For this review, take the finished solid that the model builds, in its own axes (mm). A direction names the side the tool comes from. Coordinates: 2 decimals unless noted, no trailing zeros. Order: outer loops, then holes, each group sorted by start corner. A loop starts at its lowest first (then second) coordinate and runs counter-clockwise, first axis right, second up. Notation, with made-up numbers: (26, 48.5) -> (71, 48.5) arc R34 ccw to (71, 85.5) -> close; hole circle Ø11 at (-27.5, 48.25). An arc over 180 degrees is marked (long way). Write item = value, one per line. Start each with the question number.
1) Wall thickness on probe 1 along X at (y, z) = (1.5, 0.85); probe 2 along Y at (x, z) = (-3.5, 0.7): over which ranges is each line inside the solid? List them lowest first. Write a range as [from, to].
2) Consider section C-C on y = -6. Give the boundary of the cut face in (x, z).
3) Consider section A-A on z = 1.2. Give the boundary of the cut face in (x, y).
4) Draft analysis for pull direction Y (two halves, no side actions). For faces 3 (the face through (0, 20, 1)), 4 (the face through (-9, -15, 1)), 5 (the face through (0, -16, 1)), 6 (the face through (-20, 0, 1)), state which applies: +Y half, -Y half, draft (parallel to the pull), parting line (faces both ways), or undercut.
5) Machinability: for faces 1 (the face through (-15, -9, 1)), 2 (the face through (0, -20, 1)), which of the approach directions +Z, -Z, +X, -X, +Y, -Y give a long, thin tool a straight path to every point of the face, cutting with its end or side? Answer none if there is none.
6) Insertion check: pin 1 Ø8 at (x, y) = (1, 15.5) entering from -Z. The pin has a flat end and moves straight along its axis. Give the tip position at first contact, or say it passes through.
7) Consider section B-B on x = -6. Give the boundary of the cut face in (y, z), and give its area (3 significant figures).
from build123d import *

# Parameters (mm, degrees)
F0_W     = 40
F0_H     = 40
F0_W_2   = 18
F0_H_2   = 2
F0_W_3   = 2
F0_H_3   = 18
F1_DEPTH = 3
F2_R     = 2


with BuildPart() as f1:
    # F0 (on Top) → F1 (new body)
    with BuildSketch(Plane.XY):
        Rectangle(F0_W, F0_H)
        with Locations((0, -15)):
            Rectangle(F0_W_2, F0_H_2, mode=Mode.SUBTRACT)
        with Locations((-15, 0)):
            Rectangle(F0_W_3, F0_H_3, mode=Mode.SUBTRACT)
        with Locations((15, 0)):
            Rectangle(F0_W_3, F0_H_3, mode=Mode.SUBTRACT)
    extrude(amount=F1_DEPTH)

    # F2
    f2_edges = [f1.edges().sort_by_distance(p)[0] for p in [
        (20, -20, 1.5),
        (-20, -20, 1.5),
        (-20, 20, 1.5),
        (20, 20, 1.5),
    ]]
    fillet(f2_edges, radius=F2_R)


solid = f1.part
Answer sheet:
q1.probe_1 = [-20, -16], [-14, 14], [16, 20]
q1.probe_2 = [-20, -16], [-14, 20]
q2.outline = (-20, 0) -> (-16, 0) -> (-16, 3) -> (-20, 3) -> close; (-14, 0) -> (14, 0) -> (14, 3) -> (-14, 3) -> close; (16, 0) -> (20, 0) -> (20, 3) -> (16, 3) -> close
q3.outline = (-20, -18) arc R2 ccw to (-18, -20) -> (18, -20) arc R2 ccw to (20, -18) -> (20, 18) arc R2 ccw to (18, 20) -> (-18, 20) arc R2 ccw to (-20, 18) -> close; hole (-16, -9) -> (-14, -9) -> (-14, 9) -> (-16, 9) -> close; hole (-9, -16) -> (9, -16) -> (9, -14) -> (-9, -14) -> close; hole (14, -9) -> (16, -9) -> (16, 9) -> (14, 9) -> close
q4.face_3 = +Y half
q4.face_4 = undercut
q4.face_5 = undercut
q4.face_6 = draft
q5.face_1 = +Z, -Z
q5.face_2 = +Z, -Z, +X, -X, -Y
q6.pin_1 = 0
q7.outline = (-20, 0) -> (-16, 0) -> (-16, 3) -> (-20, 3) -> close; (-14, 0) -> (20, 0) -> (20, 3) -> (-14, 3) -> close
q7.area = 114 mm2
